from build123d import *

# Parameters (mm, degrees)
SKETCH1_W                      = 600
SKETCH1_H                      = 700
BASE_FLANGE1_DEPTH             = 2.7
EDGE_FLANGE1_STRIP_W           = 14.8
EDGE_FLANGE1_STRIP_H           = 2.7
EDGE_FLANGE1_STRIP_CUT_DEPTH   = 700
EDGE_FLANGE1_STRIP_2_W         = 14.8
EDGE_FLANGE1_STRIP_2_H         = 2.7
EDGE_FLANGE1_STRIP_CUT_2_DEPTH = 700
EDGE_FLANGE1_DEPTH             = 700
EDGE_FLANGE1_BEND_DEPTH        = 700
CUT_EXTRUDE1_REACH             = 925.326
SKETCH12_W                     = 50
SKETCH12_H                     = 20
SKETCH13_W                     = 490.6
SKETCH13_H                     = 9.2
CUT_EXTRUDE2_DEPTH             = 924.476583352
CUT_EXTRUDE6_REACH             = 925.477
SKETCH17_R                     = 2
CUT_EXTRUDE7_START             = -2.7
CUT_EXTRUDE7_OUTLINE_R         = 2
CUT_EXTRUDE7_DEPTH             = 2.7
CUT_EXTRUDE10_START            = -2.7
CUT_EXTRUDE10_OUTLINE_R        = 3
CUT_EXTRUDE10_DEPTH            = 2.7


# Read off the part's stored shape, not the designer's step: Cut-Extrude7, Cut-Extrude10
# Sheet-metal steps are written as plain solids
with BuildPart() as part:
    # Sketch1 → Base-Flange1 (new body)
    with BuildSketch(Plane.XY):
        with Locations((300, 350)):
            Rectangle(SKETCH1_W, SKETCH1_H)
    extrude(amount=-BASE_FLANGE1_DEPTH)

    # Edge-Flange1 strip (across the edge) → Edge-Flange1 strip cut (cut)
    with BuildSketch(Plane(origin=(600, 0, 0), x_dir=(-1, 0, 0), z_dir=(0, 1, 0))):
        with Locations((-2.7, -1.35)):
            Rectangle(EDGE_FLANGE1_STRIP_W, EDGE_FLANGE1_STRIP_H)
    extrude(amount=EDGE_FLANGE1_STRIP_CUT_DEPTH, mode=Mode.SUBTRACT)

    # Edge-Flange1 strip 2 (across the edge) → Edge-Flange1 strip cut 2 (cut)
    with BuildSketch(Plane.XZ.offset(-700)):
        with Locations((-2.7, -1.35)):
            Rectangle(EDGE_FLANGE1_STRIP_2_W, EDGE_FLANGE1_STRIP_2_H)
    extrude(amount=EDGE_FLANGE1_STRIP_CUT_2_DEPTH, mode=Mode.SUBTRACT)

    # Edge-Flange1 section (across the edge) → Edge-Flange1 (add)
    with BuildSketch(Plane(origin=(600, 0, 0), x_dir=(-1, 0, 0), z_dir=(0, 1, 0))):
        with BuildLine():
            Line((0, 2), (0, 50.3))
            Line((0, 50.3), (2.7, 50.3))
            Line((2.7, 50.3), (2.7, 2))
            ThreePointArc((2.7, 2), (3.285786438, 0.585786438), (4.7, 0))
            Line((4.7, 0), (4.7, -2.7))
            ThreePointArc((4.7, -2.7), (1.376598128, -1.323401872), (0, 2))
        make_face()
    extrude(amount=EDGE_FLANGE1_DEPTH)

    # Edge-Flange1 section 2 (across the edge) → Edge-Flange1 bend (add)
    with BuildSketch(Plane.XZ.offset(-700)):
        with BuildLine():
            Line((0, 2), (0, 50.3))
            Line((0, 50.3), (2.7, 50.3))
            Line((2.7, 50.3), (2.7, 2))
            ThreePointArc((2.7, 2), (3.285786438, 0.585786438), (4.7, 0))
            Line((4.7, 0), (4.7, -2.7))
            ThreePointArc((4.7, -2.7), (1.376598128, -1.323401872), (0, 2))
        make_face()
    extrude(amount=EDGE_FLANGE1_BEND_DEPTH)

    # Sketch12 → Cut-Extrude1 (cut, up to next)
    with BuildSketch(Plane.XY, mode=Mode.PRIVATE) as cut_extrude1_sk1:
        with Locations((447.3, 657)):
            Rectangle(SKETCH12_W, SKETCH12_H)
    cut_extrude1_tool1 = extrude(cut_extrude1_sk1.sketch, amount=-CUT_EXTRUDE1_REACH, mode=Mode.PRIVATE) & part.part
    add(cut_extrude1_tool1.solids().sort_by_distance((447.3, 657, 0))[0], mode=Mode.SUBTRACT)

    # Sketch13 → Cut-Extrude2 (cut, through all)
    with BuildSketch(Plane(origin=(0, 0, -2.7), x_dir=(-1, 0, 0), z_dir=(0, 0, -1))):
        with Locations((-300, 4.6)):
            Rectangle(SKETCH13_W, SKETCH13_H)
    extrude(amount=-CUT_EXTRUDE2_DEPTH, mode=Mode.SUBTRACT)

    # Sketch17 → Cut-Extrude6 (cut, up to next)
    with BuildSketch(Plane(origin=(0, 0, -2.7), x_dir=(-1, 0, 0), z_dir=(0, 0, -1)), mode=Mode.PRIVATE) as cut_extrude6_sk1:
        with Locations((-560.7, 685)):
            Circle(SKETCH17_R)
    cut_extrude6_tool1 = extrude(cut_extrude6_sk1.sketch, amount=-CUT_EXTRUDE6_REACH, mode=Mode.PRIVATE) & part.part
    # Sketch17 → Cut-Extrude6 (cut, up to next)
    with BuildSketch(Plane(origin=(0, 0, -2.7), x_dir=(-1, 0, 0), z_dir=(0, 0, -1)), mode=Mode.PRIVATE) as cut_extrude6_sk2:
        with Locations((-560.7, 671.7)):
            Circle(SKETCH17_R)
    cut_extrude6_tool2 = extrude(cut_extrude6_sk2.sketch, amount=-CUT_EXTRUDE6_REACH, mode=Mode.PRIVATE) & part.part
    # Sketch17 → Cut-Extrude6 (cut, up to next)
    with BuildSketch(Plane(origin=(0, 0, -2.7), x_dir=(-1, 0, 0), z_dir=(0, 0, -1)), mode=Mode.PRIVATE) as cut_extrude6_sk3:
        with Locations((-504, 635)):
            Circle(SKETCH17_R)
    cut_extrude6_tool3 = extrude(cut_extrude6_sk3.sketch, amount=-CUT_EXTRUDE6_REACH, mode=Mode.PRIVATE) & part.part
    # Sketch17 → Cut-Extrude6 (cut, up to next)
    with BuildSketch(Plane(origin=(0, 0, -2.7), x_dir=(-1, 0, 0), z_dir=(0, 0, -1)), mode=Mode.PRIVATE) as cut_extrude6_sk4:
        with Locations((-553, 598)):
            Circle(SKETCH17_R)
    cut_extrude6_tool4 = extrude(cut_extrude6_sk4.sketch, amount=-CUT_EXTRUDE6_REACH, mode=Mode.PRIVATE) & part.part
    # Sketch17 → Cut-Extrude6 (cut, up to next)
    with BuildSketch(Plane(origin=(0, 0, -2.7), x_dir=(-1, 0, 0), z_dir=(0, 0, -1)), mode=Mode.PRIVATE) as cut_extrude6_sk5:
        with Locations((-553, 565)):
            Circle(SKETCH17_R)
    cut_extrude6_tool5 = extrude(cut_extrude6_sk5.sketch, amount=-CUT_EXTRUDE6_REACH, mode=Mode.PRIVATE) & part.part
    # Sketch17 → Cut-Extrude6 (cut, up to next)
    with BuildSketch(Plane(origin=(0, 0, -2.7), x_dir=(-1, 0, 0), z_dir=(0, 0, -1)), mode=Mode.PRIVATE) as cut_extrude6_sk6:
        with Locations((-530, 19.2)):
            Circle(SKETCH17_R)
    cut_extrude6_tool6 = extrude(cut_extrude6_sk6.sketch, amount=-CUT_EXTRUDE6_REACH, mode=Mode.PRIVATE) & part.part
    # Sketch17 → Cut-Extrude6 (cut, up to next)
    with BuildSketch(Plane(origin=(0, 0, -2.7), x_dir=(-1, 0, 0), z_dir=(0, 0, -1)), mode=Mode.PRIVATE) as cut_extrude6_sk7:
        with Locations((-471, 19.2)):
            Circle(SKETCH17_R)
    cut_extrude6_tool7 = extrude(cut_extrude6_sk7.sketch, amount=-CUT_EXTRUDE6_REACH, mode=Mode.PRIVATE) & part.part
    # Sketch17 → Cut-Extrude6 (cut, up to next)
    with BuildSketch(Plane(origin=(0, 0, -2.7), x_dir=(-1, 0, 0), z_dir=(0, 0, -1)), mode=Mode.PRIVATE) as cut_extrude6_sk8:
        with Locations((-129, 19.2)):
            Circle(SKETCH17_R)
    cut_extrude6_tool8 = extrude(cut_extrude6_sk8.sketch, amount=-CUT_EXTRUDE6_REACH, mode=Mode.PRIVATE) & part.part
    # Sketch17 → Cut-Extrude6 (cut, up to next)
    with BuildSketch(Plane(origin=(0, 0, -2.7), x_dir=(-1, 0, 0), z_dir=(0, 0, -1)), mode=Mode.PRIVATE) as cut_extrude6_sk9:
        with Locations((-70, 19.2)):
            Circle(SKETCH17_R)
    cut_extrude6_tool9 = extrude(cut_extrude6_sk9.sketch, amount=-CUT_EXTRUDE6_REACH, mode=Mode.PRIVATE) & part.part
    # Sketch17 → Cut-Extrude6 (cut, up to next)
    with BuildSketch(Plane(origin=(0, 0, -2.7), x_dir=(-1, 0, 0), z_dir=(0, 0, -1)), mode=Mode.PRIVATE) as cut_extrude6_sk10:
        with Locations((-47, 565)):
            Circle(SKETCH17_R)
    cut_extrude6_tool10 = extrude(cut_extrude6_sk10.sketch, amount=-CUT_EXTRUDE6_REACH, mode=Mode.PRIVATE) & part.part
    # Sketch17 → Cut-Extrude6 (cut, up to next)
    with BuildSketch(Plane(origin=(0, 0, -2.7), x_dir=(-1, 0, 0), z_dir=(0, 0, -1)), mode=Mode.PRIVATE) as cut_extrude6_sk11:
        with Locations((-47, 598)):
            Circle(SKETCH17_R)
    cut_extrude6_tool11 = extrude(cut_extrude6_sk11.sketch, amount=-CUT_EXTRUDE6_REACH, mode=Mode.PRIVATE) & part.part
    # Sketch17 → Cut-Extrude6 (cut, up to next)
    with BuildSketch(Plane(origin=(0, 0, -2.7), x_dir=(-1, 0, 0), z_dir=(0, 0, -1)), mode=Mode.PRIVATE) as cut_extrude6_sk12:
        with Locations((-96, 635)):
            Circle(SKETCH17_R)
    cut_extrude6_tool12 = extrude(cut_extrude6_sk12.sketch, amount=-CUT_EXTRUDE6_REACH, mode=Mode.PRIVATE) & part.part
    # Sketch17 → Cut-Extrude6 (cut, up to next)
    with BuildSketch(Plane(origin=(0, 0, -2.7), x_dir=(-1, 0, 0), z_dir=(0, 0, -1)), mode=Mode.PRIVATE) as cut_extrude6_sk13:
        with Locations((-39.3, 671.7)):
            Circle(SKETCH17_R)
    cut_extrude6_tool13 = extrude(cut_extrude6_sk13.sketch, amount=-CUT_EXTRUDE6_REACH, mode=Mode.PRIVATE) & part.part
    # Sketch17 → Cut-Extrude6 (cut, up to next)
    with BuildSketch(Plane(origin=(0, 0, -2.7), x_dir=(-1, 0, 0), z_dir=(0, 0, -1)), mode=Mode.PRIVATE) as cut_extrude6_sk14:
        with Locations((-39.3, 685)):
            Circle(SKETCH17_R)
    cut_extrude6_tool14 = extrude(cut_extrude6_sk14.sketch, amount=-CUT_EXTRUDE6_REACH, mode=Mode.PRIVATE) & part.part
    add(cut_extrude6_tool1.solids().sort_by_distance((560.7, 685, -2.7))[0], mode=Mode.SUBTRACT)
    add(cut_extrude6_tool2.solids().sort_by_distance((560.7, 671.7, -2.7))[0], mode=Mode.SUBTRACT)
    add(cut_extrude6_tool3.solids().sort_by_distance((504, 635, -2.7))[0], mode=Mode.SUBTRACT)
    add(cut_extrude6_tool4.solids().sort_by_distance((553, 598, -2.7))[0], mode=Mode.SUBTRACT)
    add(cut_extrude6_tool5.solids().sort_by_distance((553, 565, -2.7))[0], mode=Mode.SUBTRACT)
    add(cut_extrude6_tool6.solids().sort_by_distance((530, 19.2, -2.7))[0], mode=Mode.SUBTRACT)
    add(cut_extrude6_tool7.solids().sort_by_distance((471, 19.2, -2.7))[0], mode=Mode.SUBTRACT)
    add(cut_extrude6_tool8.solids().sort_by_distance((129, 19.2, -2.7))[0], mode=Mode.SUBTRACT)
    add(cut_extrude6_tool9.solids().sort_by_distance((70, 19.2, -2.7))[0], mode=Mode.SUBTRACT)
    add(cut_extrude6_tool10.solids().sort_by_distance((47, 565, -2.7))[0], mode=Mode.SUBTRACT)
    add(cut_extrude6_tool11.solids().sort_by_distance((47, 598, -2.7))[0], mode=Mode.SUBTRACT)
    add(cut_extrude6_tool12.solids().sort_by_distance((96, 635, -2.7))[0], mode=Mode.SUBTRACT)
    add(cut_extrude6_tool13.solids().sort_by_distance((39.3, 671.7, -2.7))[0], mode=Mode.SUBTRACT)
    add(cut_extrude6_tool14.solids().sort_by_distance((39.3, 685, -2.7))[0], mode=Mode.SUBTRACT)

    # Cut-Extrude7 outline → Cut-Extrude7 (cut)
    with BuildSketch(Plane.XY.offset(CUT_EXTRUDE7_START)):
        with Locations((352, 508)):
            Circle(CUT_EXTRUDE7_OUTLINE_R)
        with Locations((580, 505)):
            Circle(CUT_EXTRUDE7_OUTLINE_R)
        with Locations((580, 525)):
            Circle(CUT_EXTRUDE7_OUTLINE_R)
        with Locations((342, 508)):
            Circle(CUT_EXTRUDE7_OUTLINE_R)
    extrude(amount=CUT_EXTRUDE7_DEPTH, mode=Mode.SUBTRACT)

    # Cut-Extrude10 outline → Cut-Extrude10 (cut)
    with BuildSketch(Plane.XY.offset(CUT_EXTRUDE10_START)):
        with Locations((219.3, 541.9)):
            Circle(CUT_EXTRUDE10_OUTLINE_R)
        with Locations((380.8, 121.9)):
            Circle(CUT_EXTRUDE10_OUTLINE_R)
        with Locations((219.3, 261.9)):
            Circle(CUT_EXTRUDE10_OUTLINE_R)
        with Locations((219.3, 201.9)):
            Circle(CUT_EXTRUDE10_OUTLINE_R)
        with Locations((380.8, 181.9)):
            Circle(CUT_EXTRUDE10_OUTLINE_R)
        with Locations((380.8, 241.9)):
            Circle(CUT_EXTRUDE10_OUTLINE_R)
        with Locations((380.8, 301.9)):
            Circle(CUT_EXTRUDE10_OUTLINE_R)
        with Locations((219.3, 141.9)):
            Circle(CUT_EXTRUDE10_OUTLINE_R)
        with Locations((219.3, 81.9)):
            Circle(CUT_EXTRUDE10_OUTLINE_R)
        with Locations((380.8, 81.9)):
            Circle(CUT_EXTRUDE10_OUTLINE_R)
        with Locations((219.3, 321.9)):
            Circle(CUT_EXTRUDE10_OUTLINE_R)
        with Locations((380.8, 361.9)):
            Circle(CUT_EXTRUDE10_OUTLINE_R)
        with Locations((219.3, 381.9)):
            Circle(CUT_EXTRUDE10_OUTLINE_R)
        with Locations((380.8, 421.9)):
            Circle(CUT_EXTRUDE10_OUTLINE_R)
        with Locations((219.3, 441.9)):
            Circle(CUT_EXTRUDE10_OUTLINE_R)
        with Locations((380.8, 481.9)):
            Circle(CUT_EXTRUDE10_OUTLINE_R)
        with Locations((219.3, 501.9)):
            Circle(CUT_EXTRUDE10_OUTLINE_R)
        with Locations((380.8, 541.9)):
            Circle(CUT_EXTRUDE10_OUTLINE_R)
    extrude(amount=CUT_EXTRUDE10_DEPTH, mode=Mode.SUBTRACT)


solid = part.part
Read the model definition and answer for the solid it produces. Units are mm, in the model's axes. A direction names the side the tool comes from. Round coordinates to 2 decimals unless told otherwise and drop trailing zeros. Order: outer loops, then holes, each group sorted by start corner. A loop starts at its lowest first (then second) coordinate and runs counter-clockwise, first axis right, second up. Notation, with made-up numbers: (60.25, 46.5) - (81.25, 46.5) arc R29 ccw to (81.25, 72.5) - close; hole circle Ø1 at (-34, 21.25). An arc over 180 degrees is marked (long way). Use one line per item in the form item = value. Start each with the question number.
(1) The part is cut by section C-C (y = 230.5). Give the vertices of the cut face in (x, z).
(2) The part is cut by section D-D (x = 189). Give the vertices of the cut face in (y, z).
(3) For faces 1 (the face through (597.3, 345, 26)), 2 (the face through (301, 700, -2)), determine the directions among +Z, -Z, +X, -X, +Y, -Y from which every point of the face is accessible in a straight line to the end or side of a thin tool.
(4) The part is cut by section A-A (z = 21). Give the vertices of the cut face in (x, y).
(5) Find the intervals of material crossed by line 1 along X through (y, z) = (367.5, 12); line 2 along Z through (x, y) = (558.5, 269); line 3 along X through (y, z) = (505, -1.3), in increasing order. Write a range as from..to.
(6) The part is cut by section B-B (x = 443). Give the vertices of the cut face in (y, z).
(7) Determine the mould class of faces 3 (the face through (600, 345, 26)), 4 (the face through (296, 355, 0)), 5 (the face through (585, 0, -2)) for opening direction X: +X half, -X half, draft (parallel to the pull), parting line (faces both ways), or undercut.
(8) Flat-ended cylindrical pins translate along their axes: pin 1 Ø3.5 at (x, y) = (352, 508) entering from -Z; pin 2 Ø5 at (x, y) = (39.3, 685) entering from +Z; pin 3 Ø3 at (y, z) = (6, -1.5) entering from +X; pin 4 Ø0.8 at (y, z) = (659, -2) entering from +X. Find the tip coordinate at first contact, or state that the pin passes through.
Checked values:
q1.outline = (0, 2) arc R4.7 ccw to (4.7, -2.7) - (595.3, -2.7) arc R4.7 ccw to (600, 2) - (600, 50.3) - (597.3, 50.3) - (597.3, 2) arc R2 cw to (595.3, 0) - (4.7, 0) arc R2 cw to (2.7, 2) - (2.7, 50.3) - (0, 50.3) - close
q2.outline = (9.2, -2.7) - (700, -2.7) - (700, 0) - (9.2, 0) - close
q3.face_1 = +Z, +Y, -Y
q3.face_2 = +Z, -Z, +X, -X, +Y
q4.outline = (0, 0) - (2.7, 0) - (2.7, 700) - (0, 700) - close; (597.3, 0) - (600, 0) - (600, 700) - (597.3, 700) - close
q5.line_1 = 0..2.7, 597.3..600
q5.line_2 = -2.7..0
q5.line_3 = 1.35..578, 582..598.65
q6.outline = (9.2, -2.7) - (647, -2.7) - (647, 0) - (9.2, 0) - close; (667, -2.7) - (700, -2.7) - (700, 0) - (667, 0) - close
q7.face_3 = +X half
q7.face_4 = undercut
q7.face_5 = draft
q8.pin_1 = through
q8.pin_2 = 0
q8.pin_3 = 599.55
q8.pin_4 = 598.32
